Build history of the part. All positions in model axes, mm. A direction names the side the tool comes from. Round coordinates to 2 decimals unless told otherwise and drop trailing zeros. Write each loop counter-clockwise with the first axis right and the second up, starting at its lowest first coordinate (ties: lowest second). Pieces come first, ordered by that corner, then holes. Notation, with made-up numbers: M -35,82.5 L -12,82.5 A12 ccw -12,86.5 Z; hole C 41.5,29 d1. An arc over 180 degrees is marked long. Use a Markdown table: item, result.
from build123d import *

# Parameters (mm, degrees)
SKETCH2_W           = 1000
SKETCH2_H           = 10
EXTRUDE_THIN1_DEPTH = 20
SKETCH4_W           = 10.725253094
SKETCH4_H           = 20
BOSS_EXTRUDE1_DEPTH = 1


with BuildPart() as part:
    # Sketch2 → Extrude-Thin1 (new body)
    with BuildSketch(Plane.XY):
        with Locations((0, 5)):
            Rectangle(SKETCH2_W, SKETCH2_H)
    extrude(amount=EXTRUDE_THIN1_DEPTH)

    # Sketch4 → Boss-Extrude1 (add)
    with BuildSketch(Plane(origin=(0, 10, 0), x_dir=(1, 0, 0), z_dir=(0, 1, 0))):
        with Locations((0, -10)):
            Rectangle(SKETCH4_W, SKETCH4_H)
    extrude(amount=BOSS_EXTRUDE1_DEPTH)


solid = part.part
Q1. Drop flat-ended pins along their axis: P1, Ø10, axis at x = -350, z = 10, coming from the +Y side; P2, Ø4, axis at x = 353, z = 8.5, coming from the -Y side. Give the stop position or say it passes through.
Response values:
| item | result |
|---|---|
| P1 | stops at y = 10 |
| P2 | stops at y = 0 |
Q2. Cut at A-A on z = 3.5. Give the cut face in (x, y).
Response values:
| item | result |
|---|---|
| outline | M -500,0 L 500,0 L 500,10 L 5.36,10 L 5.36,11 L -5.36,11 L -5.36,10 L -500,10 Z |
Q3. Cut at B-B on x = -109.5. Give the cut face in (y, z).
Response values:
| item | result |
|---|---|
| outline | M 0,0 L 10,0 L 10,20 L 0,20 Z |
Q4. Which spindle directions (+Z, -Z, +X, -X, +Y, -Y) get a long thin tool onto all of the face, cutting with end or side? Do faces 1 (the flat face through (-256, 10, 10)), 2 (the flat face through (-7, 0, 10)), 3 (the flat face through (249, 10, 10)). Say none if no direction does.
Response values:
| item | result |
|---|---|
| face 1 | +Z, -Z, -X, +Y |
| face 2 | +Z, -Z, +X, -X, -Y |
| face 3 | +Z, -Z, +X, +Y |
Q5. Drill centre lines: L1, parallel to Y at x = -89.5, z = 8; L2, parallel to X at y = 10.25, z = 11. Where is each one in solid material? Low to high.
Response values:
| item | result |
|---|---|
| L1 | y = 0 to 10 |
| L2 | x = -5.36 to 5.36 |
